Source: CAD feature listing. Evaluate the final solid. Frame: model axes, mm. Face numbers are marked on the shaded views. Coordinates: 2 decimals unless noted, no trailing zeros. Write each loop counter-clockwise with the first axis right and the second up, starting at its lowest first coordinate (ties: lowest second). Pieces come first, ordered by that corner, then holes. Notation, with made-up numbers: (44.25, 78.5) -> (85.25, 78.5) arc R14 cw to (85.25, 93.5) -> close; hole circle Ø3 at (63.25, -29). An arc over 180 degrees is marked (long way). Write item = value, one per line.
from build123d import *

# Parameters (mm, degrees)
F1_DEPTH = 50.8


# Not quite as in the source:
# - a feature names something its author has since deleted; it is built from what else it names


with BuildPart() as f1:
    # F0 (on Front) → F1 (new body)
    with BuildSketch(Plane.XZ):
        with BuildLine():
            Line((7.9375, -1.9304), (10.8458, 14.2875))
            ThreePointArc((10.8458, 14.2875), (0, 9.3006063571), (-10.8458, 14.2875))
            Line((-10.8458, 14.2875), (-7.9375, -1.9304))
            Line((-7.9375, -1.9304), (-5.3791059517, -1.9304))
            ThreePointArc((-5.3791059517, -1.9304), (-0.9797026298, 5.6304003194), (5.715, 0))
            ThreePointArc((5.715, 0), (5.6304003194, -0.9797026298), (5.3791059517, -1.9304))
            Line((5.3791059517, -1.9304), (7.9375, -1.9304))
        make_face()
    extrude(amount=F1_DEPTH)


solid = f1.part
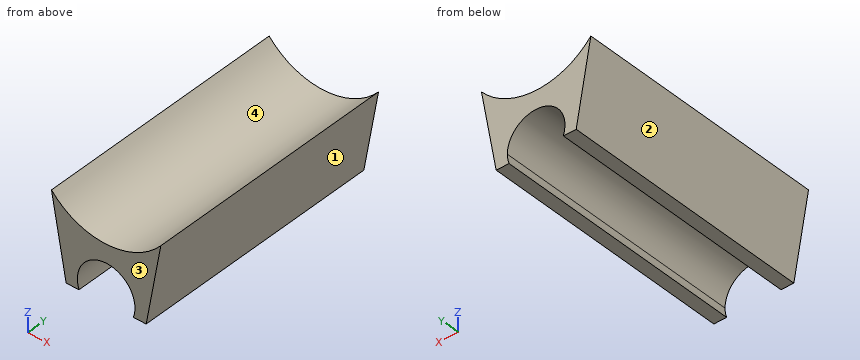
1) Cut plane A-A, the plane y = -20.5. Output: boundary loops of the cut face in (x, z) (1 decimal), and give its area (3 significant figures).
Answer block:
outline = (-10.8, 14.3) -> (-7.9, -1.9) -> (-5.4, -1.9) arc R5.7 cw (long way) to (5.4, -1.9) -> (7.9, -1.9) -> (10.8, 14.3) arc R14.3 cw to start
area = 157 mm2
2) Cut plane C-C, the plane x = 0. Output: boundary loops of the cut face in (y, z) (3 decimals), and give its area (3 significant figures).
Answer block:
outline = (-50.8, 5.715) -> (0, 5.715) -> (0, 9.301) -> (-50.8, 9.301) -> close
area = 182 mm2
3) First-contact query: pin 1 Ø2 at (y, z) = (-45.5, 4.5) entering from +X; pin 2 Ø3 at (y, z) = (-29.5, 6.5) entering from +X; pin 3 Ø5 at (y, z) = (-8.5, 5.5) entering from -X. Flat tips, straight axial feed; report the tip coordinate or a pass-through.
Answer block:
pin_1 = 9.27
pin_2 = 9.72
pin_3 = -9.72
4) Pull-direction query (X, two-part tool) for the marked faces 1, 2, 3 and 4; classes: +X half, -X half, draft (parallel to the pull), parting line (faces both ways), or undercut.
Answer block:
face_1 = +X half
face_2 = -X half
face_3 = draft
face_4 = undercut
5) Cut plane D-D, the plane z = 3.75. Output: boundary loops of the cut face in (x, y), and give its area (3 significant figures).
Answer block:
outline = (-8.96, -50.8) -> (-4.31, -50.8) -> (-4.31, 0) -> (-8.96, 0) -> close; (4.31, -50.8) -> (8.96, -50.8) -> (8.96, 0) -> (4.31, 0) -> close
area = 472 mm2
6) Material intervals for probe 1 along Z at (x, y) = (0, -26) (3 decimals); probe 2 along X at (y, z) = (-14.5, 4); probe 3 along X at (y, z) = (-21, 11.5), sorted ascending. Write a range as [from, to].
Answer block:
probe_1 = [5.715, 9.301]
probe_2 = [-9, -4.08], [4.08, 9]
probe_3 = [-10.35, -7.62], [7.62, 10.35]
